```python
from build123d import *

# Parameters (mm, degrees)
SKETCH2_R           = 40.08124111
BOSS_EXTRUDE2_DEPTH = 20
SKETCH1_W           = 5
SKETCH1_H           = 3
CUT_EXTRUDE1_DEPTH  = 8
BOSS_EXTRUDE3_DEPTH = 5


with BuildPart() as part:
    # Sketch2 → Boss-Extrude2 (new body)
    with BuildSketch(Plane(origin=(0, 0, 0), x_dir=(1, 0, 0), z_dir=(0, 1, 0))):
        with Locations((0, 15)):
            Circle(SKETCH2_R)
    extrude(amount=BOSS_EXTRUDE2_DEPTH)

    # Sketch1 → Cut-Extrude1 (cut)
    with BuildSketch(Plane(origin=(0, 0, 0), x_dir=(1, 0, 0), z_dir=(0, 1, 0))):
        with Locations((0, -4.5)):
            Rectangle(SKETCH1_W, SKETCH1_H)
        with Locations((0, -11.5)):
            Rectangle(SKETCH1_W, SKETCH1_H)
        with Locations((0, 2.5)):
            Rectangle(SKETCH1_W, SKETCH1_H)
        with Locations((0, 9.5)):
            Rectangle(SKETCH1_W, SKETCH1_H)
        with Locations((0, 16.5)):
            Rectangle(SKETCH1_W, SKETCH1_H)
        with Locations((0, 23.5)):
            Rectangle(SKETCH1_W, SKETCH1_H)
    extrude(amount=CUT_EXTRUDE1_DEPTH, mode=Mode.SUBTRACT)

    # Sketch3 → Boss-Extrude3 (add)
    with BuildSketch(Plane(origin=(0, 20, 0), x_dir=(1, 0, 0), z_dir=(0, 1, 0))):
        Polygon((0, 53.367433342), (-2.5, 26.790245023), (2.5, 26.790245023), align=None)
    extrude(amount=BOSS_EXTRUDE3_DEPTH)


solid = part.part
```
Verification items for the finished model (mm, model axes). A direction names the side the tool comes from. Give positions to 0.01 mm unless a question says otherwise; leave off trailing zeros. Order: outer loops, then holes, each group sorted by start corner. A loop starts at its lowest first (then second) coordinate and runs counter-clockwise, first axis right, second up. Notation, with made-up numbers: M 65,-22.75 L 115,-22.75 A18 ccw 115,10.25 Z; hole C 59,38.25 d11. An arc over 180 degrees is marked long. Answer in a Markdown table with one row per item. Add a question column.
Item 1: Section check B-B, the plane y = 23.25. Enter the section's corners in (x, z), and give its area (3 significant figures).
Item 2: Section check C-C, the plane x = 8. Enter the section's corners in (y, z).
Item 3: Section check A-A, the plane z = -29.5. Enter the section's corners in (x, y), and give its area (3 significant figures).
Item 4: Tool access check on faces 5 (the flat face through (-1.233, 22.465, -40.265)), 6 (the flat face through (2.5, 4, 5)). Record the directions out of +Z, -Z, +X, -X, +Y, -Y that give a thin tool (end or side, any length) a straight path to the whole face; none if there is none.
Item 5: Scan lines: probe 1 along Y at (x, z) = (23.5, -42.5); probe 2 along X at (y, z) = (17, 12); probe 3 along X at (y, z) = (19.75, -44). Record each from-to range of solid material in increasing order. Write a range as from..to.
Item 6: Section check D-D, the plane y = 12.5. Enter the section's corners in (x, z), and give its area (3 significant figures).
Item 7: Mould release check, pull along Z, two halves, no side actions. Record for faces 1 (the flat face through (0, 25, -37)), 2 (the flat face through (0, 4, -25)), 3 (the flat face through (0, 8, 11)), 4 (the flat face through (1.267, 22.465, -39.893)): released by +Z, released by -Z, zero draft, split by the parting line, or undercut.
Item 8: Gauge pin test, flat ends, axial feed: pin 1 (1.5 mm diameter, centred on x = -0.5, y = 4.5, fed in from -Z); pin 2 (4 mm diameter, centred on y = 5, z = -30.5, fed in from +X); pin 3 (4 mm diameter, centred on x = 1, y = 2, fed in from +Z). Record the tip position at first contact, or that the pin passes through.
Filled sheet:
| question | item | result |
|---|---|---|
| 1 | outline | M -2.5,-26.79 L 0,-53.37 L 2.5,-26.79 Z |
| 1 | area | 66.4 mm^2 |
| 2 | outline | M 0,-54.27 L 20,-54.27 L 20,24.27 L 0,24.27 Z |
| 3 | outline | M -37.37,0 L 37.37,0 L 37.37,20 L 2.25,20 L 2.25,25 L -2.25,25 L -2.25,20 L -37.37,20 Z |
| 3 | area | 1,520 mm^2 |
| 4 | face 5 | -Z, -X, +Y |
| 4 | face 6 | -Y |
| 5 | probe 1 | y = 0..20 |
| 5 | probe 2 | x = -29.62..29.62 |
| 5 | probe 3 | x = -27.67..27.67 |
| 6 | outline | C 0,-15 d80.16 |
| 6 | area | 5,050 mm^2 |
| 7 | face 1 | zero draft |
| 7 | face 2 | undercut |
| 7 | face 3 | undercut |
| 7 | face 4 | released by -Z |
| 8 | pin 1 | stops at z = -55.08 |
| 8 | pin 2 | stops at x = 37.74 |
| 8 | pin 3 | stops at z = 25.08 |
